Autodesk Inventor part; units mm, degrees
ref_plane "Work Plane1" through (-203.2, 0, 0) normal (-0.0012, 0, 1) x (1, 0, 0.0012)
ref_plane "Work Plane3" through (-22.225, 0, -152.6256) normal (0, 0, -1) x (-1, 0, 0)
ref_plane "YZ Plane" through (0, 0, 0) normal (1, 0, 0) x (0, 1, 0)
sketch "Sketch1" plane through (0, 0, 0) normal (0, 1, 0) x (-1, 0, 0)
  line L0 (304.8, -139.7) -> (203.2, -152.4)
  line L1 (304.8, -12.7) -> (203.2, 0)
  line L2 (304.8, -12.7) -> (304.8, -139.7)
  arc A0 (25.4, 0) -> (0, -25.4) centre (22.225, -22.225) ccw
  line L3 (203.2, 0) -> (25.4, 0)
  arc A1 (0, -127) -> (25.4, -152.4) centre (22.225, -130.175) ccw
  line L4 (203.2, -152.4) -> (25.4, -152.4)
  line L5 (0, -127) -> (0, -25.4)
  point P0 (0, 0)
  point P1 (203.2, -12.7)
  point P2 (203.2, -139.7)
  point P3 (101.6, -12.7)
  point P4 (101.6, -139.7)
  point P5 (101.6, -152.4)
  point P6 (0, -139.7)
  dimension "d8" = 12.7
  dimension "d12" = 101.6
  dimension "d13" = 127
extrude "Extrusion1" add sketch "Sketch1" against normal blind 25.4
sketch "Sketch2" plane through (0, 0, 0) normal (0, 1, 0) x (1, 0, 0)
  line L0 (-25.4, 0) -> (-203.2, 0)
  line L1 (-203.2, 152.4) -> (-25.4, 152.4)
  line L2 (-203.2, 12.7) -> (-101.6, 12.7)
  line L3 (-101.6, 12.7) -> (-101.6, 139.7)
  line L4 (-101.6, 139.7) -> (-203.2, 139.7)
  line L5 (-203.2, 139.7) -> (-203.2, 12.7)
  line L6 (-209.55, 6.35) -> (-95.25, 6.35)
  line L7 (-95.25, 6.35) -> (-95.25, 146.05)
  line L8 (-95.25, 146.05) -> (-209.55, 146.05)
  line L9 (-209.55, 146.05) -> (-209.55, 6.35)
  point P0 (0, 0)
  point P1 (-203.2, 6.35)
  dimension "d23" = 12.7
  dimension "d24" = 101.6
  dimension "d25" = 127
  dimension "d26" = 6.35
  dimension "d27" = 6.35
  dimension "d28" = 114.3
  dimension "d29" = 139.7
extrude "Extrusion2" add sketch "Sketch2" along normal blind 6.35
ref_plane "Work Plane1" through (-203.2, 0, 0) normal (-0.0012, 0, 1) x (1, 0, 0.0012)
sketch "Sketch7" plane through (-203.2, 0, 0) normal (-0.0012, 0, 1) x (1, 0, 0.0012)
  line L0 (0, 0) -> (0, -25.4)
  line L1 (0, -25.4) -> (-101.6158, -25.4)
  circle A0 centre (-50.8, -12.7) radius 6.35
  point P0 (203.1998, 0)
  dimension "d41" = 50.8
  dimension "d43" = 12.7
  dimension "d44" = 12.7
extrude "Extrusion4" cut sketch "Sketch7" against normal blind 152.4
ref_plane "Work Plane3" through (-22.225, 0, -152.6256) normal (0, 0, -1) x (-1, 0, 0)
sketch "Sketch11" plane through (0, 0, 0) normal (0, 1, 0) x (1, 0, 0)
  line L0 (-95.25, 0) -> (-25.654, 0)
  line L1 (-25.654, 0) -> (-25.654, 30.48)
  line L2 (-25.654, 30.48) -> (-95.25, 30.48)
  line L3 (-95.25, 30.48) -> (-95.25, 0)
  line L4 (-95.25, 6.35) -> (-95.25, 146.05)
  line L5 (-95.25, 152.4) -> (-25.654, 152.4)
  line L6 (-25.654, 152.4) -> (-25.654, 121.92)
  line L7 (-25.654, 121.92) -> (-95.25, 121.92)
  line L8 (-95.25, 121.92) -> (-95.25, 152.4)
  point P0 (0, 0)
  dimension "d59" = 69.596
  dimension "d60" = 30.48
  dimension "d61" = 69.596
  dimension "d62" = 30.48
extrude "Extrusion7" cut sketch "Sketch11" against normal blind 14.732
sketch "Sketch12" plane through (0, 6.35, 0) normal (0, 1, 0) x (1, 0, 0)
  line L0 (-203.2, 22.5806) -> (-203.2, 76.9366)
  line L1 (-203.2, 76.9366) -> (-209.55, 76.9366)
  line L2 (-209.55, 76.9366) -> (-209.55, 22.5806)
  line L3 (-209.55, 76.9366) -> (-203.2, 76.9366)
  line L4 (-203.2, 76.9366) -> (-203.2, 6.35)
  line L5 (-203.2, 6.35) -> (-209.55, 6.35)
  line L6 (-209.55, 6.35) -> (-209.55, 76.9366)
  point P0 (0, 0)
  point P1 (-203.2, 12.7)
  point P2 (-209.55, 6.35)
  point P3 (-209.55, 12.7)
  dimension "d67" = 9.8806
  dimension "d68" = 6.35
  dimension "d69" = 54.356
extrude "Extrusion9" cut sketch "Sketch12" against normal blind 6.35
properties part number "RC_Chassis"
Source: CAD feature listing. Evaluate the final solid. Frame: model axes, mm. A direction names the side the tool comes from. Give positions to 0.01 mm unless a question says otherwise; leave off trailing zeros. Order: outer loops, then holes, each group sorted by start corner. A loop starts at its lowest first (then second) coordinate and runs counter-clockwise, first axis right, second up.
(1) Section query A-A (x = -51.5). Return the cut outline in (y, z), plus the area to 3 significant figures.
(2) Material intervals for line 1 along X through (y, z) = (-7.5, -23); line 2 along X through (y, z) = (1, -105); line 3 along Z through (x, y) = (-103, -7), sorted ascending.
(3) Access query for faces 1 (the face through (-61, -14.732, -15)), 2 (the face through (-209.55, 3, -112)), 3 (the face through (-152, 3, -139.7)), 4 (the face through (0, -13, -77)), 5 (the face through (-61, -14.732, -137)). Directions: +Z, -Z, +X, -X, +Y, -Y. A direction counts if a zero-diameter tool reaches every point of the face in a straight line with its end or side. Return the directions, or none.
(4) Pull-direction query (Z, two-part tool) for faces 6 (the face through (-199, 0, -75)), 7 (the face through (-203.2, 3, -10)), 8 (the face through (-254.71, -20.99, -6.44)); classes: +Z half, -Z half, draft (parallel to the pull), parting line (faces both ways), or undercut.
(5) Section query B-B (y = 3). Return the cut outline in (x, z), plus the area to 3 significant figures.
(6) Section query C-C (x = -188). Return the cut outline in (y, z), plus the area to 3 significant figures.
(7) Contact query for flat-ended pins moving along their axis: P1, Ø8, axis at x = -151.5, z = -85, coming from the +Y side; P2, Ø4.5, axis at x = -67.5, y = -6, coming from the +Z side; P3, Ø6.5, axis at y = -9.5, z = -77.5, coming from the +X side. Output: stop coordinate, or through.
(8) Section query D-D (x = -232). Return the cut outline in (y, z).
Outcome:
1. outline: (-25.4, -152.4) - (-14.73, -152.4) - (-14.73, -121.92) - (0, -121.92) - (0, -30.48) - (-14.73, -30.48) - (-14.73, 0) - (-25.4, 0) - close
1. area: 2,970 mm2
2. line 1: x = -304.8 to -257.62, -250.33 to -95.25, -25.65 to 0.21
2. line 2: x = -209.55 to -203.2, -101.6 to -95.25
2. line 3: z = -152.4 to 0
3. face 1: +Z, +Y
3. face 2: +Z, -Z, -X, +Y
3. face 3: +Y
3. face 4: +X, +Y, -Y
3. face 5: -Z, +Y
4. face 6: undercut
4. face 7: draft
4. face 8: +Z half
5. outline: (-209.55, -146.05) - (-95.25, -146.05) - (-95.25, -6.35) - (-203.2, -6.35) - (-203.2, -12.7) - (-101.6, -12.7) - (-101.6, -139.7) - (-203.2, -139.7) - (-203.2, -76.94) - (-209.55, -76.94) - close
5. area: 2,620 mm2
6. outline: (-25.4, -152.4) - (0, -152.4) - (0, -146.05) - (6.35, -146.05) - (6.35, -139.7) - (0, -139.7) - (0, -12.7) - (6.35, -12.7) - (6.35, -6.35) - (0, -6.35) - (0, 0) - (-25.4, 0) - close
6. area: 3,950 mm2
7. P1: stops at y = 0
7. P2: stops at z = -30.48
7. P3: stops at x = 0
8. outline: (-25.4, -148.8) - (0, -148.8) - (0, -3.6) - (-25.4, -3.6) - close
